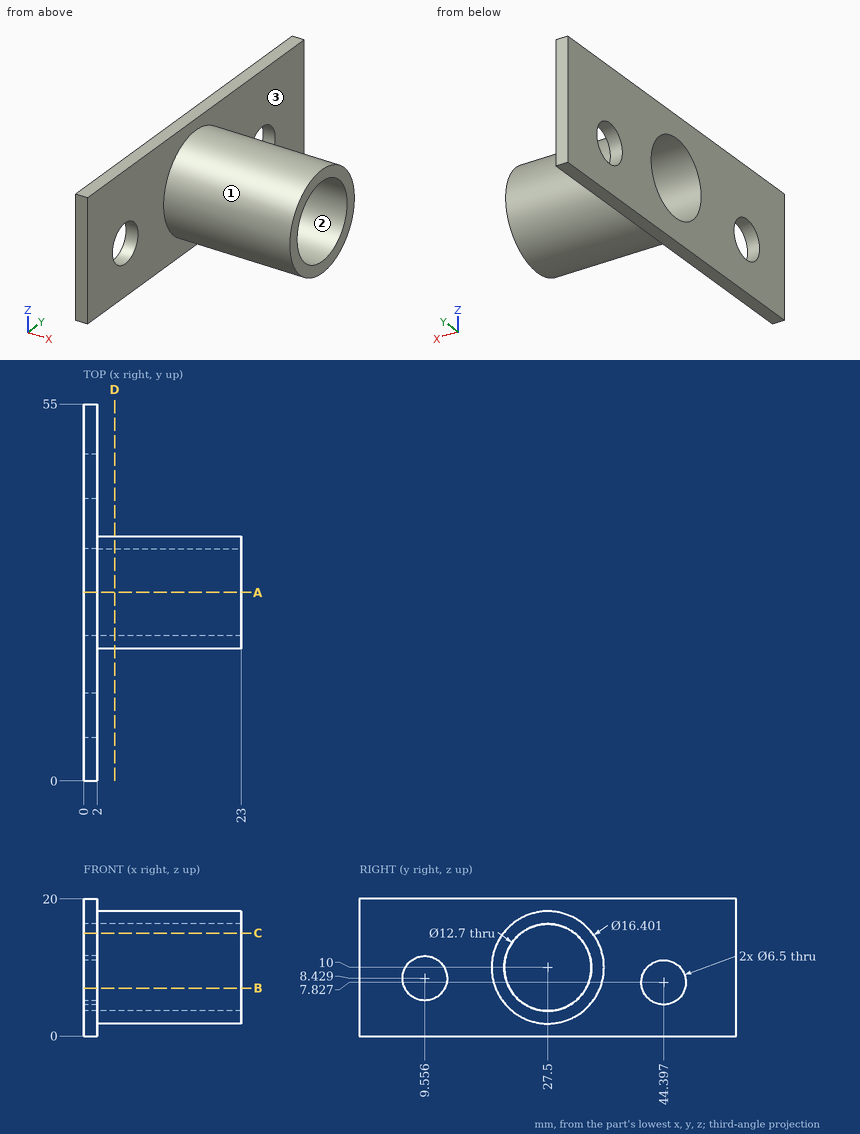
Verification items for this drawing (mm, ordinates from the low corner). Give positions to 0.01 mm unless a question says otherwise; leave off trailing zeros. Loops run counter-clockwise (first coordinate to the right, second up) from the corner with the lowest first, then second, coordinate; pieces in that order, holes last. Notation, with made-up numbers: M -28.5,86 L -10.5,86 A29 ccw -10.5,116 Z; hole C 29.25,-6 d5. An arc over 180 degrees is marked long. Answer as a JSON object with one key per item and string values. Group by question number.
Item 1: Sectioned sample at B-B on z = 7. Record the boundary of the cut face in (x, y) (1 decimal).
Item 2: Sectioned sample at A-A on y = 27.5. Record the boundary of the cut face in (x, z).
Item 3: Material ranges on L1, parallel to Y at x = 18.5, z = 10.25 (1 decimal); L2, parallel to X at y = 4.5, z = 1.25; L3, parallel to Y at x = 3, z = 6, recorded low to high.
Item 4: Sectioned sample at D-D on x = 4.5. Record the boundary of the cut face in (y, z).
Item 5: Mould release check, pull along Y, two halves, no side actions. Record for the marked faces 1, 2 and 3: pulls with the +Y half, pulls with the -Y half, needs draft (parallel to the pull), parting line crosses it, or undercut.
Item 6: Sectioned sample at C-C on z = 15. Record the boundary of the cut face in (x, y) (1 decimal), plus the area to 3 significant figures.
Item 7: Gauge pin test, flat ends, axial feed: pin 1 (5 mm diameter, centred on x = 15, z = 4.5, fed in from +Y); pin 2 (12 mm diameter, centred on x = 14, z = 2.5, fed in from +Y); pin 3 (2 mm diameter, centred on x = 8.5, z = 15, fed in from -Y). Record the tip position at first contact, or that the pin passes through.
Findings below:
{
 "1": {"outline": "M 0,0 L 2,0 L 2,6.6 L 0,6.6 Z; M 0,12.5 L 2,12.5 L 2,19.9 L 23,19.9 L 23,21.9 L 0,21.9 Z; M 0,33.1 L 23,33.1 L 23,35.1 L 2,35.1 L 2,41.3 L 0,41.3 Z; M 0,47.5 L 2,47.5 L 2,55 L 0,55 Z"},
 "2": {"outline": "M 0,0 L 2,0 L 2,1.8 L 23,1.8 L 23,3.65 L 0,3.65 Z; M 0,16.35 L 23,16.35 L 23,18.2 L 2,18.2 L 2,20 L 0,20 Z"},
 "3": {"L1": "19.3 to 21.2, 33.8 to 35.7", "L2": "0 to 2", "L3": "20.34 to 22.57, 32.43 to 34.66"},
 "4": {"outline": "C 27.5,10 d16.4; hole C 27.5,10 d12.7"},
 "5": {"face 1": "parting line crosses it", "face 2": "undercut", "face 3": "needs draft"},
 "6": {"outline": "M 0,0 L 2,0 L 2,21 L 23,21 L 23,23.6 L 0,23.6 Z; M 0,31.4 L 23,31.4 L 23,34 L 2,34 L 2,55 L 0,55 Z", "area": "203 mm2"},
 "7": {"pin 1": "y = 35.13", "pin 2": "y = 35.56", "pin 3": "y = 20.34"}
}
